Autodesk Inventor part; units mm, degrees
ref_plane "YZ Plane" through (0, 0, 0) normal (1, 0, 0) x (0, 1, 0)
ref_plane "XZ Plane" through (0, 0, 0) normal (0, 1, 0) x (-1, 0, 0)
ref_plane "XY Plane" through (0, 0, 0) normal (0, 0, 1) x (1, 0, 0)
sketch "草圖1" plane through (0, 0, 0) normal (0, 0, 1) x (1, 0, 0)
  line L0 (-5, -5) -> (5, -5)
  line L1 (5, -5) -> (5, 5)
  line L2 (5, 5) -> (-5, 5)
  line L3 (-5, 5) -> (-5, -5)
  line L4 (-5, -5) -> (5, 5) construction
  line L5 (5, -5) -> (-5, 5) construction
  line L6 (-7, 7) -> (7, 7)
  line L7 (7, 7) -> (7, -7)
  line L8 (7, -7) -> (-7, -7)
  line L9 (-7, -7) -> (-7, 7)
  point P0 (0, 0)
  dimension "d0" = 10
  dimension "d1" = 10
  dimension "d2" = 2
extrude "擠出1" add sketch "草圖1" along normal blind 10
sketch "草圖2" plane through (-7, 7, 0) normal (0, 1, 0) x (1, 0, 0)
  line L0 (2, -10) -> (12, -10)
  line L1 (12, 0) -> (2, 0)
  line L2 (4, -10) -> (9, -10)
  line L3 (9, -10) -> (9, 0)
  line L4 (9, 0) -> (4, 0)
  line L5 (4, 0) -> (4, -10)
  line L6 (14, 0) -> (14, -10)
  point P0 (7, 0)
  dimension "d5" = 5
  dimension "d6" = 5
extrude "擠出2" add sketch "草圖2" along normal blind 15
sketch "草圖3" plane through (0, 0, 10) normal (0, 0, 1) x (1, 0, 0)
  line L0 (-7, 7) -> (-3, 7)
  line L1 (-7, 7) -> (8.7829, 7)
  line L2 (8.7829, 7) -> (8.7829, 28.6907)
  line L3 (8.7829, 28.6907) -> (-7, 28.6907)
  line L4 (-7, 28.6907) -> (-7, 7)
  point P0 (0, 0)
extrude "擠出3" cut sketch "草圖3" against normal blind 2.5
sketch "草圖4" plane through (0, 0, 0) normal (0, 0, -1) x (-1, 0, 0)
  line L0 (-2, 7) -> (-7, 7)
  line L1 (-3.5131, 7) -> (8.3925, 7)
  line L2 (8.3925, 7) -> (8.3925, 27.422)
  line L3 (8.3925, 27.422) -> (-3.5131, 27.422)
  line L4 (-3.5131, 27.422) -> (-3.5131, 7)
  point P0 (0, 0)
extrude "擠出4" cut sketch "草圖4" against normal blind 2.5
fillet "圓角2" radius 2.5 4 edges at (-3, 14.5, 7.5) (2, 14.5, 7.5) (2, 14.5, 2.5) (-3, 14.5, 2.5)
fillet "圓角3" radius 2.5 3 edges at (-3, 22, 5) (-2.2678, 22, 6.7678) (-0.5, 22, 7.5)
properties part number "軸滑塊"
Verification items for the finished model (mm, model axes). A direction names the side the tool comes from. Round coordinates to 2 decimals unless told otherwise and drop trailing zeros. Write each loop counter-clockwise with the first axis right and the second up, starting at its lowest first coordinate (ties: lowest second). Pieces come first, ordered by that corner, then holes. Notation, with made-up numbers: (53, 27) -> (62, 27) arc R12 ccw to (62, 48) -> close; hole circle Ø1 at (2.25, 34). An arc over 180 degrees is marked (long way). Write each question's results on one line, items separated by ' | '.
Q1. Access from +Z, -Z, +X, -X, +Y, -Y to the whole of each face (thin tool, end or side, straight path). Record for faces 1 (the face through (-2, 13, 3)), 2 (the face through (1, 13, 7)), 3 (the face through (-2, 13, 7)), 4 (the face through (1, 13, 3)), 5 (the face through (0, -5, 5)).
Derived:
face 1: -Z, -X, +Y | face 2: +Z, +X, +Y | face 3: +Z, -X, +Y | face 4: -Z, +X, +Y | face 5: +Z, -Z
Q2. Sectioned sample at B-B, the plane z = 8.75. Record the boundary of the cut face in (x, y), and give its area (3 significant figures).
Derived:
outline: (-7, -7) -> (7, -7) -> (7, 7) -> (-7, 7) -> close; hole (-5, -5) -> (5, -5) -> (5, 5) -> (-5, 5) -> close | area: 96.0 mm²
Q3. Sectioned sample at A-A, the plane y = -3. Record the boundary of the cut face in (x, z).
Derived:
outline: (-7, 0) -> (-5, 0) -> (-5, 10) -> (-7, 10) -> close; (5, 0) -> (7, 0) -> (7, 10) -> (5, 10) -> close
Q4. Draft check along Y on faces 6 (the face through (1.5, 7, 2.7)), 7 (the face through (0, 5, 5)), 8 (the face through (-7, 0, 5)), 9 (the face through (5, 0, 5)). Enter one of: released by +Y, released by -Y, zero draft, split by the parting line, or undercut.
Derived:
face 6: released by +Y | face 7: undercut | face 8: zero draft | face 9: undercut
Q5. Go/stop test with flat-tipped pins: pin 1 Ø5 at (x, z) = (3.5, 6) entering from +Y; pin 2 Ø5 at (x, z) = (1, 9) entering from +Y; pin 3 Ø4 at (x, y) = (-2, 18.5) entering from -Z. Record where each tip stops, or that it passes through.
Derived:
pin 1: stops at y = 21.4 | pin 2: stops at y = 21.26 | pin 3: stops at z = 2.5
Q6. Thickness scan on probe 1 along X at (y, z) = (-4.25, 2); probe 2 along Z at (x, y) = (-0.5, 11). Record the ranges inside material, lowest first.
Derived:
probe 1: x = -7 to -5, 5 to 7 | probe 2: z = 2.5 to 7.5
